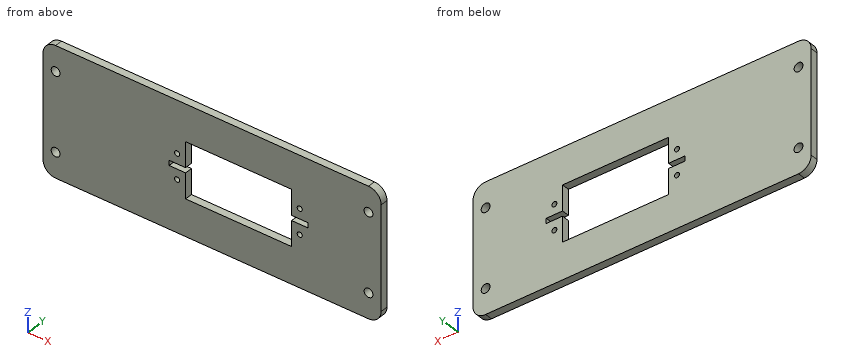
```python
from build123d import *

# Parameters (mm, degrees)
SKETCH_1_W          = 134
SKETCH_1_H          = 51
EXTRUDE_1_DEPTH     = 3
CUT_EXTRUDE_1_REACH = 73.751
SKETCH_2_R          = 1.75
CUT_EXTRUDE_2_REACH = 73.751
SKETCH_3_R          = 1
FILLET_1_R          = 5


with BuildPart() as part:
    # 스케치1 → 보스-돌출1 (new body)
    with BuildSketch(Plane(origin=(0, 0, 0), x_dir=(1, 0, 0), z_dir=(0, 1, 0))):
        Rectangle(SKETCH_1_W, SKETCH_1_H)
    extrude(amount=EXTRUDE_1_DEPTH)

    # 스케치2 → 컷-돌출1 (cut, up to next)
    with BuildSketch(Plane(origin=(0, 3, 0), x_dir=(1, 0, 0), z_dir=(0, 1, 0)), mode=Mode.PRIVATE) as cut_extrude_1_sk1:
        with Locations(Location((-62, 15.5, 0), (0, 0, 270))):
            Circle(SKETCH_2_R)
    cut_extrude_1_tool1 = extrude(cut_extrude_1_sk1.sketch, amount=-CUT_EXTRUDE_1_REACH, mode=Mode.PRIVATE) & part.part
    # 스케치2 → 컷-돌출1 (cut, up to next)
    with BuildSketch(Plane(origin=(0, 3, 0), x_dir=(1, 0, 0), z_dir=(0, 1, 0)), mode=Mode.PRIVATE) as cut_extrude_1_sk2:
        with Locations(Location((-62, -15.5, 0), (0, 0, 270))):
            Circle(SKETCH_2_R)
    cut_extrude_1_tool2 = extrude(cut_extrude_1_sk2.sketch, amount=-CUT_EXTRUDE_1_REACH, mode=Mode.PRIVATE) & part.part
    # 스케치2 → 컷-돌출1 (cut, up to next)
    with BuildSketch(Plane(origin=(0, 3, 0), x_dir=(1, 0, 0), z_dir=(0, 1, 0)), mode=Mode.PRIVATE) as cut_extrude_1_sk3:
        with Locations(Location((62, 15.5, 0), (0, 0, 270))):
            Circle(SKETCH_2_R)
    cut_extrude_1_tool3 = extrude(cut_extrude_1_sk3.sketch, amount=-CUT_EXTRUDE_1_REACH, mode=Mode.PRIVATE) & part.part
    # 스케치2 → 컷-돌출1 (cut, up to next)
    with BuildSketch(Plane(origin=(0, 3, 0), x_dir=(1, 0, 0), z_dir=(0, 1, 0)), mode=Mode.PRIVATE) as cut_extrude_1_sk4:
        with Locations(Location((62, -15.5, 0), (0, 0, 270))):
            Circle(SKETCH_2_R)
    cut_extrude_1_tool4 = extrude(cut_extrude_1_sk4.sketch, amount=-CUT_EXTRUDE_1_REACH, mode=Mode.PRIVATE) & part.part
    add(cut_extrude_1_tool1.solids().sort_by_distance((-62, 3, -15.5))[0], mode=Mode.SUBTRACT)
    add(cut_extrude_1_tool2.solids().sort_by_distance((-62, 3, 15.5))[0], mode=Mode.SUBTRACT)
    add(cut_extrude_1_tool3.solids().sort_by_distance((62, 3, -15.5))[0], mode=Mode.SUBTRACT)
    add(cut_extrude_1_tool4.solids().sort_by_distance((62, 3, 15.5))[0], mode=Mode.SUBTRACT)

    # 스케치3 → 컷-돌출2 (cut, up to next)
    with BuildSketch(Plane(origin=(0, 3, 0), x_dir=(1, 0, 0), z_dir=(0, 1, 0)), mode=Mode.PRIVATE) as cut_extrude_2_sk1:
        with Locations(Location((-13.85, 5, 0), (0, 0, 270))):
            Circle(SKETCH_3_R)
    cut_extrude_2_tool1 = extrude(cut_extrude_2_sk1.sketch, amount=-CUT_EXTRUDE_2_REACH, mode=Mode.PRIVATE) & part.part
    # 스케치3 → 컷-돌출2 (cut, up to next)
    with BuildSketch(Plane(origin=(0, 3, 0), x_dir=(1, 0, 0), z_dir=(0, 1, 0)), mode=Mode.PRIVATE) as cut_extrude_2_sk2:
        with Locations(Location((-13.85, -5, 0), (0, 0, 270))):
            Circle(SKETCH_3_R)
    cut_extrude_2_tool2 = extrude(cut_extrude_2_sk2.sketch, amount=-CUT_EXTRUDE_2_REACH, mode=Mode.PRIVATE) & part.part
    # 스케치3 → 컷-돌출2 (cut, up to next)
    with BuildSketch(Plane(origin=(0, 3, 0), x_dir=(1, 0, 0), z_dir=(0, 1, 0)), mode=Mode.PRIVATE) as cut_extrude_2_sk3:
        with Locations(Location((34.75, 5, 0), (0, 0, 270))):
            Circle(SKETCH_3_R)
    cut_extrude_2_tool3 = extrude(cut_extrude_2_sk3.sketch, amount=-CUT_EXTRUDE_2_REACH, mode=Mode.PRIVATE) & part.part
    # 스케치3 → 컷-돌출2 (cut, up to next)
    with BuildSketch(Plane(origin=(0, 3, 0), x_dir=(1, 0, 0), z_dir=(0, 1, 0)), mode=Mode.PRIVATE) as cut_extrude_2_sk4:
        with Locations(Location((34.75, -5, 0), (0, 0, 270))):
            Circle(SKETCH_3_R)
    cut_extrude_2_tool4 = extrude(cut_extrude_2_sk4.sketch, amount=-CUT_EXTRUDE_2_REACH, mode=Mode.PRIVATE) & part.part
    # 스케치3 → 컷-돌출2 (cut, up to next)
    with BuildSketch(Plane(origin=(0, 3, 0), x_dir=(1, 0, 0), z_dir=(0, 1, 0)), mode=Mode.PRIVATE) as cut_extrude_2_sk5:
        Polygon((-10.5, 11), (31.5, 11), (31.5, 1), (38, 1), (38, -1), (31.5, -1), (31.5, -11), (-10.5, -11), (-10.5, -1), (-17, -1), (-17, 1), (-10.5, 1), align=None)
    cut_extrude_2_tool5 = extrude(cut_extrude_2_sk5.sketch, amount=-CUT_EXTRUDE_2_REACH, mode=Mode.PRIVATE) & part.part
    add(cut_extrude_2_tool1.solids().sort_by_distance((-13.85, 3, -5))[0], mode=Mode.SUBTRACT)
    add(cut_extrude_2_tool2.solids().sort_by_distance((-13.85, 3, 5))[0], mode=Mode.SUBTRACT)
    add(cut_extrude_2_tool3.solids().sort_by_distance((34.75, 3, -5))[0], mode=Mode.SUBTRACT)
    add(cut_extrude_2_tool4.solids().sort_by_distance((34.75, 3, 5))[0], mode=Mode.SUBTRACT)
    add(cut_extrude_2_tool5.solids().sort_by_distance((10.5, 3, 0))[0], mode=Mode.SUBTRACT)

    # 필렛1
    fillet_1_edges = [part.edges().sort_by_distance(p)[0] for p in [
        (67, 1.5, 25.5),
        (-67, 1.5, 25.5),
        (-67, 1.5, -25.5),
        (67, 1.5, -25.5),
    ]]
    fillet(fillet_1_edges, radius=FILLET_1_R)


solid = part.part
```
Could you check a few things on this model? Use its own coordinates, in mm. Coordinates: 2 decimals unless noted, no trailing zeros. Order: outer loops, then holes, each group sorted by start corner. A loop starts at its lowest first (then second) coordinate and runs counter-clockwise, first axis right, second up. Notation, with made-up numbers: M 80.5,73 L 122.5,73 A34 cw 122.5,108 Z; hole C 21.25,85 d11. An arc over 180 degrees is marked long. Use one line per item in the form item = value. Start each with the question number.
1. Suppose I cut it at B-B on x = 8.5. Write out the boundary of the cut face in (y, z), then the cut area to 3 significant figures.
2. Suppose I cut it at C-C on z = -8.5. Write out the boundary of the cut face in (x, y).
3. Suppose I cut it at D-D on y = 1.2. Count the separate pieces of the cut face and the enclosed holes in it, then the cut area to 3 significant figures.
4. Please list where these lines run through material, in increasing order: line 1 (X direction, y = 1.1, z = -5); line 2 (X direction, y = 1.65, z = 15.5); line 3 (Z direction, x = 26.5, y = 0.75).
5. Suppose I cut it at A-A on z = 15.5. Write out the boundary of the cut face in (x, y), then the cut area to 3 significant figures.
Geometry says:
q1.outline = M 0,-25.5 L 3,-25.5 L 3,-11 L 0,-11 Z; M 0,11 L 3,11 L 3,25.5 L 0,25.5 Z
q1.area = 87.0 mm^2
q2.outline = M -67,0 L -10.5,0 L -10.5,3 L -67,3 Z; M 31.5,0 L 67,0 L 67,3 L 31.5,3 Z
q3.separate_pieces = 1
q3.enclosed_holes = 9
q3.area = 5,810 mm^2
q4.line_1 = -67 to -14.85, -12.85 to -10.5, 31.5 to 33.75, 35.75 to 67
q4.line_2 = -67 to -63.75, -60.25 to 60.25, 63.75 to 67
q4.line_3 = -25.5 to -11, 11 to 25.5
q5.outline = M -67,0 L -63.75,0 L -63.75,3 L -67,3 Z; M -60.25,0 L 60.25,0 L 60.25,3 L -60.25,3 Z; M 63.75,0 L 67,0 L 67,3 L 63.75,3 Z
q5.area = 381 mm^2
